Drawing for the job (mm, zero at the part's lowest x, y, z). Give positions to 0.01 mm unless a question says otherwise; leave off trailing zeros. Order: outer loops, then holes, each group sorted by start corner. A loop starts at its lowest first (then second) coordinate and runs counter-clockwise, first axis right, second up. Notation, with made-up numbers: (23, 36.25) - (75, 36.25) arc R11 cw to (75, 44.25) - close; hole circle Ø10 at (36.25, 47). An arc over 180 degrees is marked (long way). One line per item, written item: value.
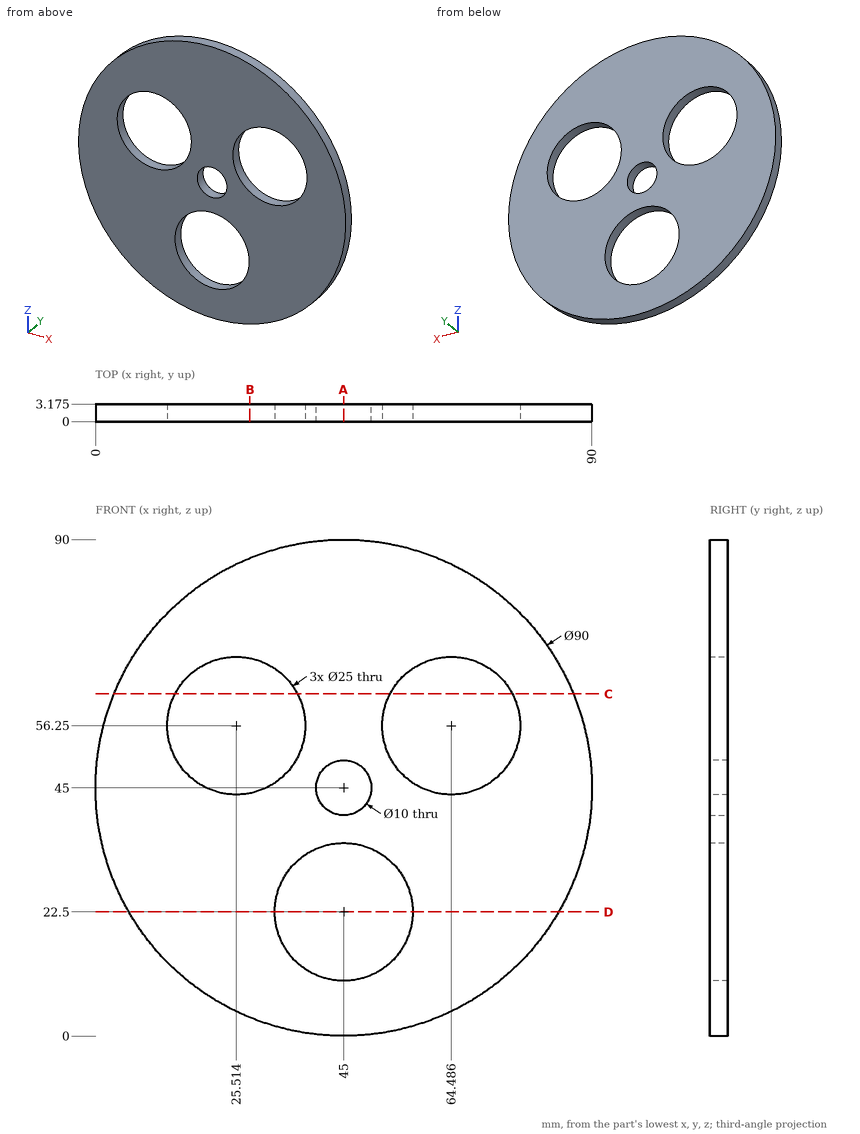
1) Cut at D-D, the plane z = 22.5. Give the cut face in (x, y) (1 decimal).
Outcome:
outline: (6, 0) - (32.5, 0) - (32.5, 3.2) - (6, 3.2) - close; (57.5, 0) - (84, 0) - (84, 3.2) - (57.5, 3.2) - close
2) Drill centre lines: line 1 along X through (y, z) = (0.8, 51); line 2 along X through (y, z) = (2.25, 45) (1 decimal); line 3 along X through (y, z) = (0.75, 47) (1 decimal). Where is each one in solid material? Low to high. Write a range as from..to.
Outcome:
line 1: x = 0.4..14.17, 36.86..53.14, 75.83..89.6
line 2: x = 0..20.1, 31..40, 50..59, 69.9..90
line 3: x = 0..17.1, 33.9..40.4, 49.6..56.1, 72.9..90
3) Cut at A-A, the plane x = 45. Give the cut face in (y, z) (1 decimal), then the cut area to 3 significant figures.
Outcome:
outline: (0, 0) - (3.2, 0) - (3.2, 10) - (0, 10) - close; (0, 35) - (3.2, 35) - (3.2, 40) - (0, 40) - close; (0, 50) - (3.2, 50) - (3.2, 90) - (0, 90) - close
area: 175 mm^2
4) Cut at B-B, the plane x = 28. Give the cut face in (y, z) (1 decimal), then the cut area to 3 significant figures.
Outcome:
outline: (0, 3.3) - (3.2, 3.3) - (3.2, 44) - (0, 44) - close; (0, 68.5) - (3.2, 68.5) - (3.2, 86.7) - (0, 86.7) - close
area: 187 mm^2
5) Pin check, flat tips, straight feed: pin 1 (1 mm diameter, centred on x = 71, y = 2.5, fed in from -Z); pin 2 (1.5 mm diameter, centred on x = 74, y = 0.5, fed in from -Z). Stop position of each tip, or through.
Outcome:
pin 1: stops at z = 7.92
pin 2: stops at z = 9.97
6) Cut at C-C, the plane z = 62. Give the cut face in (x, y) (1 decimal), then the cut area to 3 significant figures.
Outcome:
outline: (3.3, 0) - (14.4, 0) - (14.4, 3.2) - (3.3, 3.2) - close; (36.6, 0) - (53.4, 0) - (53.4, 3.2) - (36.6, 3.2) - close; (75.6, 0) - (86.7, 0) - (86.7, 3.2) - (75.6, 3.2) - close
area: 124 mm^2
